The model under review builds one solid part; all positions refer to its coordinate system, in mm. A direction names the side the tool comes from. Round coordinates to 2 decimals unless told otherwise and drop trailing zeros. Loops run counter-clockwise (first coordinate to the right, second up) from the corner with the lowest first, then second, coordinate; pieces in that order, holes last. Notation, with made-up numbers: (12, -24.5) -> (60, -24.5) arc R20 cw to (60, -16.5) -> close; hole circle Ø1 at (4.5, 6). An arc over 180 degrees is marked (long way). Return JSON: item names as keys, results as strings. Group by question number.
Autodesk Inventor part; units mm, degrees
ref_plane "YZ Plane" through (0, 0, 0) normal (1, 0, 0) x (0, 1, 0)
ref_plane "XZ Plane" through (0, 0, 0) normal (0, 1, 0) x (-1, 0, 0)
ref_plane "XY Plane" through (0, 0, 0) normal (0, 0, 1) x (1, 0, 0)
sketch "Sketch1" plane through (0, 0, 0) normal (1, 0, 0) x (0, 1, 0)
  circle A0 centre (17, 0) radius 15 construction
  line L0 (42, 0) -> (42, 18)
  line L1 (42, 18) -> (10.539, 18)
  line L2 (10.539, 18) -> (0, 7.461)
  line L3 (0, 7.461) -> (0, 0)
  line L4 (42, 0) -> (0, 0) construction
  line L5 (42, 0) -> (42, -18)
  line L6 (42, -18) -> (10.539, -18)
  line L7 (10.539, -18) -> (0, -7.461)
  line L8 (0, -7.461) -> (0, 0)
  line L9 (0, 15.5075) -> (0, -16.6542) construction
  dimension "d0" = 30
  dimension "d1" = 17
  dimension "d2" = 25
  dimension "d3" = 18
  dimension "d5" = 135
extrude "Extrusion1" add sketch "Sketch1" along normal blind 15
sketch "Sketch2" plane through (15, 0, 0) normal (1, 0, 0) x (0, 0, -1)
  circle A0 centre (0, 17) radius 15
  point P0 (0, 0)
  dimension "d8" = 30
  dimension "d9" = 17
extrude "Extrusion2" cut sketch "Sketch2" against normal blind 10
sketch "Sketch3" plane through (5, 17, 0) normal (1, 0, 0) x (0, 0, -1)
  circle A0 centre (0, 0) radius 7.5
  point P0 (0, -17)
  dimension "d12" = 15
extrude "Extrusion3" cut sketch "Sketch3" against normal blind 4
sketch "Sketch4" plane through (1, 17, 0) normal (1, 0, 0) x (0, 0, -1)
  circle A0 centre (0, 0) radius 7.5
  circle A1 centre (0, 0) radius 2.25
  point P0 (0, -17)
  dimension "d15" = 4.5
extrude "Extrusion4" cut sketch "Sketch4" against normal up to next contours A1
sketch "Sketch5" plane through (0, 0, 0) normal (-1, 0, 0) x (0, 0, 1)
  circle A0 centre (0, 17) radius 2.25
  circle A1 centre (0, 17) radius 12 construction
  point P0 (0, 0)
  point P1 (-12, 17)
  point P2 (12, 17)
  dimension "d18" = 24
hole "Hole1" at (0, 17, -12) at (0, 17, 12) direction (1, 0, 0) diameter 2.459 end through all counterbore diameter 6 counterbore depth 3.5
sketch "Sketch6" plane through (0, 42, 18) normal (0, 1, 0) x (1, 0, 0)
  line L0 (0, 18) -> (15, 18) construction
  line L1 (15, 10.539) -> (15, 25.461) construction
  line L2 (15, 36) -> (15, 0) construction
  point P0 (9, 5.5)
  point P1 (9, 30.5)
  dimension "d26" = 12.5
  dimension "d27" = 6
hole "Hole2" at (9, 42, 12.5) at (9, 42, -12.5) direction (0, -1, 0) diameter 4.917 depth 5 tip angle 118
fillet "Fillet1" radius 17 2 edges at (7.5, 0, -7.461) (7.5, 0, 7.461)
properties part number "Porte_encodeur"
1. We need section C-C, the plane x = 12.5. Write out the cut boundary in (y, z), then the cut area to 3 significant figures.
2. We need section B-B, the plane x = 4.5. Write out the cut boundary in (y, z), then the cut area to 3 significant figures.
3. For P1, Ø4, axis at y = 17, z = 12, coming from the +X side; P2, Ø18, axis at y = 17, z = 0, coming from the -X side; P3, Ø1, axis at x = 6.5, y = 10, coming from the -Z side; P4, Ø6, axis at x = 6, z = 9.5, coming from the -Y side, all flat-tipped, find the tip position at first contact; note any pin that passes through.
4. Draft analysis for pull direction X (two halves, no side actions). For faces 1 (the face through (9.29, 35.78, 12.19)), 2 (the face through (7.338, 39.465, 10.688)), 3 (the face through (0, 21, 0)), 4 (the face through (7.4, 7.8, -15.26)), state which applies: pulls with the +X half, pulls with the -X half, needs draft (parallel to the pull), parting line crosses it, or undercut.
5. Tool access review of faces 5 (the face through (1.77, 19.93, 11.35)), 6 (the face through (3.028, 24.436, 0.976)), 7 (the face through (4.26, 16.631, 13.173)): name each direction out of +Z, -Z, +X, -X, +Y, -Y from which nothing blocks a thin tool from reaching the whole face with its end or side.
6. We need section A-A, the plane y = 17. Give the number of separate pieces and of enclosed holes in the cut face, then the cut area to 3 significant figures.
7. We need section D-D, the plane z = 3. Write out the cut boundary in (x, y), then the cut area to 3 significant figures.
8. Wall thickness on line 1 (Z direction, x = 9, y = 38.95); line 2 (Y direction, x = 12.25, z = 0); line 3 (Y direction, x = 3.9, z = 0): over which ranges is each line inside the solid? List them lowest first.
Check sheet entries:
{
 "1": {"outline": "(0, -0.42) arc R17 ccw to (4.98, -12.44) -> (10.54, -18) -> (42, -18) -> (42, 18) -> (10.54, 18) -> (4.98, 12.44) arc R17 ccw to (0, 0.42) -> close; hole circle Ø30 at (17, 0)", "area": "682 mm²"},
 "2": {"outline": "(0, -0.42) arc R17 ccw to (4.98, -12.44) -> (10.54, -18) -> (42, -18) -> (42, 18) -> (10.54, 18) -> (4.98, 12.44) arc R17 ccw to (0, 0.42) -> close; hole circle Ø15 at (17, 0); hole circle Ø2.46 at (17, -12); hole circle Ø2.46 at (17, 12)", "area": "1,200 mm²"},
 "3": {"P1": "stops at x = 5", "P2": "stops at x = 0", "P3": "stops at z = -17.96", "P4": "stops at y = 1.12"},
 "4": {"face 1": "undercut", "face 2": "undercut", "face 3": "pulls with the -X half", "face 4": "needs draft"},
 "5": {"face 5": "-X", "face 6": "+X", "face 7": "+X, -X"},
 "6": {"separate pieces": "4", "enclosed holes": "0", "area": "126 mm²"},
 "7": {"outline": "(0, 0.2) -> (15, 0.2) -> (15, 2.3) -> (5, 2.3) -> (5, 10.13) -> (1, 10.13) -> (1, 23.87) -> (5, 23.87) -> (5, 31.7) -> (15, 31.7) -> (15, 42) -> (0, 42) -> close", "area": "278 mm²"},
 "8": {"line 1": "z = -18 to -14.96, -10.04 to 10.04, 14.96 to 18", "line 2": "y = 0 to 2, 32 to 42", "line 3": "y = 0 to 9.5, 24.5 to 42"}
}
